Source: CAD feature listing. Evaluate the final solid. Frame: model axes, mm. Face numbers are marked on the shaded views. A direction names the side the tool comes from. Give positions to 0.01 mm unless a question says otherwise; leave off trailing zeros. Write each loop counter-clockwise with the first axis right and the second up, starting at its lowest first coordinate (ties: lowest second). Pieces come first, ordered by that corner, then holes. Notation, with made-up numbers: (71, -36.75) -> (104, -36.75) arc R8 ccw to (104, -22.75) -> close; hole circle Ø3 at (76, 33.5). An arc over 180 degrees is marked (long way). Write item = value, one per line.
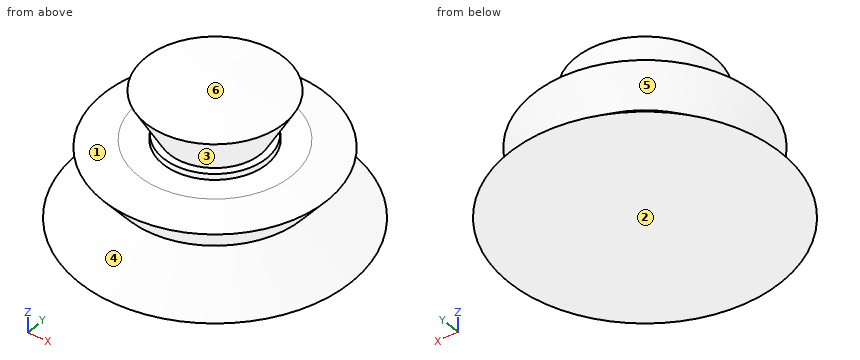
from build123d import *


with BuildPart() as f1:
    # F0 (on Front) → F1 (revolve)
    with BuildSketch(Plane.XZ):
        Polygon((27.708905, 51.024929), (0, 55.75572), (0, 0), (54.404069, 0), (34.805086, 15.881931), (44.796481, 28.211742), (18.247325, 34.129258), align=None)
    revolve(axis=Axis((0, 0, 27.87786), (0, 0, -1)))

    # F2 (on Right) → F3 (revolve, cut)
    with BuildSketch(Plane.YZ):
        Polygon((-20.794654, 31.364221), (-20.621512, 33.615056), (-31.009976, 31.364221), align=None)
    revolve(axis=Axis((0, 0, 28.211742), (0, 0, -1)), mode=Mode.SUBTRACT)


solid = f1.part
1) Contact query for flat-ended pins moving along their axis: pin 1 (1.5 mm diameter, centred on x = -21, z = 25, fed in from +Y); pin 2 (1 mm diameter, centred on y = 20.5, z = 11.5, fed in from +X); pin 3 (4 mm diameter, centred on y = 26, z = 27.5, fed in from -X). Output: stop coordinate, or through.
Computed:
pin_1 = 37.41
pin_2 = 35.37
pin_3 = -37.74
2) Access query for the marked faces 5 and 6. Directions: +Z, -Z, +X, -X, +Y, -Y. A direction counts if a zero-diameter tool reaches every point of the face in a straight line with its end or side. Return the directions, or none.
Computed:
face_5 = none
face_6 = +Z
3) Material intervals for L1, parallel to Z at x = -29, y = -0.5; L2, parallel to Z at x = 39, y = 11.5; L3, parallel to Z at x = -9.5, y = -24, sorted ascending.
Computed:
L1 = 0 to 31.36
L2 = 0 to 11.14, 23.11 to 29.13
L3 = 0 to 31.36, 47.64 to 51.35
4) Cut plane B-B (z = 5). Return the cut outline in (x, y), then the cut area to 3 significant figures.
Computed:
outline = circle Ø96.47 at (0, 0)
area = 7,310 mm²
5) Cut plane A-A (z = 11). Return the cut outline in (x, y), then the cut area to 3 significant figures.
Computed:
outline = circle Ø81.66 at (0, 0)
area = 5,240 mm²
6) Draft query along Z for the marked faces 1, 2, 3 and 4. Return one class per face: pulls with the +Z half, pulls with the -Z half, needs draft (parallel to the pull), parting line crosses it, or undercut.
Computed:
face_1 = pulls with the +Z half
face_2 = pulls with the -Z half
face_3 = undercut
face_4 = undercut
